```python
from build123d import *

# Parameters (mm, degrees)
F0_W     = 50.8
F0_H     = 76.2
F1_DEPTH = 152.4
F2_R     = 5.08
F3_T     = -4.7752
F4_R     = 6.35
F5_DEPTH = 4.7752


with BuildPart() as f1:
    # F0 (on Right) → F1 (new body)
    with BuildSketch(Plane.YZ):
        with Locations((25.4, 38.1)):
            Rectangle(F0_W, F0_H)
    extrude(amount=F1_DEPTH)

    # F2
    f2_edges = [f1.edges().sort_by_distance(p)[0] for p in [
        (76.2, 0, 76.2),
        (76.2, 50.8, 76.2),
        (76.2, 0, 0),
        (76.2, 50.8, 0),
    ]]
    fillet(f2_edges, radius=F2_R)

    # F3
    f3_openings = [f1.faces().sort_by_distance(p)[0] for p in [
        (152.4, 25.4, 38.1),
        (0, 25.4, 38.1),
    ]]
    offset(amount=F3_T, openings=f3_openings)

    # F4 (on face) → F5 (cut, through all)
    with BuildSketch(Plane.XZ):
        with Locations((38.1, 38.1)):
            Circle(F4_R)
        with Locations((114.3, 38.1)):
            Circle(F4_R)
    extrude(amount=-F5_DEPTH, mode=Mode.SUBTRACT)


solid = f1.part
```
Build history of the part. All positions in model axes, mm. A direction names the side the tool comes from. Round coordinates to 2 decimals unless told otherwise and drop trailing zeros. Order: outer loops, then holes, each group sorted by start corner. A loop starts at its lowest first (then second) coordinate and runs counter-clockwise, first axis right, second up. Notation, with made-up numbers: (10, 10) - (50, 10) arc R16 ccw to (50, 38) - close; hole circle Ø11 at (-29, -28.5). An arc over 180 degrees is marked (long way). Use a Markdown table: item, result.
1) Flat gauge pin, fed straight in: pin 1 Ø8 at (y, z) = (18.5, 12.5) entering from -X. Where does the tip first touch, or does it go through?
Recorded:
| item | result |
|---|---|
| pin 1 | passes through |
2) Tool access for faces 1 (the face through (75, 46.025, 38)), 2 (the face through (33.06, 2.35, 34.24)), 3 (the face through (77.267, 49.272, 1.449)): list every direction of +Z, -Z, +X, -X, +Y, -Y with a clear straight run to the whole face (end or side of a thin tool).
Recorded:
| item | result |
|---|---|
| face 1 | +X, -X |
| face 2 | -Y |
| face 3 | -Z, +X, -X, +Y |
3) Pull direction X, two halves, no side cores. Call faces 4 (the face through (0, 48, 39)), 5 (the face through (109.26, 2.35, 34.24)), 6 (the face through (75, 25, 4.775)), 7 (the face through (152.4, 48, 39)): pulls with the +X half, pulls with the -X half, needs draft (parallel to the pull), parting line crosses it, or undercut.
Recorded:
| item | result |
|---|---|
| face 4 | pulls with the -X half |
| face 5 | undercut |
| face 6 | needs draft |
| face 7 | pulls with the +X half |
4) Saw through at D-D on z = 38.1. Write the cut outline in (x, y).
Recorded:
| item | result |
|---|---|
| outline | (0, 0) - (31.75, 0) - (31.75, 4.78) - (0, 4.78) - close; (0, 46.02) - (152.4, 46.02) - (152.4, 50.8) - (0, 50.8) - close; (44.45, 0) - (107.95, 0) - (107.95, 4.78) - (44.45, 4.78) - close; (120.65, 0) - (152.4, 0) - (152.4, 4.78) - (120.65, 4.78) - close |
5) Saw through at A-A on y = 24. Write the cut outline in (x, z).
Recorded:
| item | result |
|---|---|
| outline | (0, 0) - (152.4, 0) - (152.4, 4.78) - (0, 4.78) - close; (0, 71.42) - (152.4, 71.42) - (152.4, 76.2) - (0, 76.2) - close |
6) Saw through at B-B on x = 63. Write the cut outline in (y, z).
Recorded:
| item | result |
|---|---|
| outline | (0, 5.08) arc R5.08 ccw to (5.08, 0) - (45.72, 0) arc R5.08 ccw to (50.8, 5.08) - (50.8, 71.12) arc R5.08 ccw to (45.72, 76.2) - (5.08, 76.2) arc R5.08 ccw to (0, 71.12) - close; hole (4.78, 5.08) arc R0.3 ccw to (5.08, 4.78) - (45.72, 4.78) arc R0.3 ccw to (46.02, 5.08) - (46.02, 71.12) arc R0.3 ccw to (45.72, 71.42) - (5.08, 71.42) arc R0.3 ccw to (4.78, 71.12) - close |
7) Wall check: L1, parallel to Y at x = 12, z = 62.5; L2, parallel to Z at x = 25, y = 18.5; L3, parallel to Z at x = 38.1, y = 1.8. Give the ranges that are in metal, low to high.
Recorded:
| item | result |
|---|---|
| L1 | y = 0 to 4.78, 46.02 to 50.8 |
| L2 | z = 0 to 4.78, 71.42 to 76.2 |
| L3 | z = 1.2 to 31.75, 44.45 to 75 |
8) Saw through at C-C on z = 58.5. Write the cut outline in (x, y), and give its area (3 significant figures).
Recorded:
| item | result |
|---|---|
| outline | (0, 0) - (152.4, 0) - (152.4, 4.78) - (0, 4.78) - close; (0, 46.02) - (152.4, 46.02) - (152.4, 50.8) - (0, 50.8) - close |
| area | 1,460 mm² |
